Study the drawing (mm; zero at the part's minimum x, y, z) and answer. A direction names the side the tool comes from. Round coordinates to 2 decimals unless told otherwise and drop trailing zeros. Order: outer loops, then holes, each group sorted by start corner. A loop starts at its lowest first (then second) coordinate and runs counter-clockwise, first axis right, second up. Notation, with made-up numbers: (-29.5, 51.5) - (11.5, 51.5) arc R17 ccw to (11.5, 55.5) - close; hole circle Ø9 at (50.5, 43). An arc over 180 degrees is marked (long way). Put each result on its own line as item: value. Start each with the question number.
Q1. Section C-C on x = 3.5 is taken. Give the vertices of the cut face in (y, z) (3 decimals).
Q2. Section B-B on y = 17 is taken. Give the vertices of the cut face in (x, z), then the cut area to 3 significant figures.
Q3. Each of these flat-tipped pins is pushed along its axis until it touches: pin 1 Ø8 at (x, z) = (7, 14) entering from +Y; pin 2 Ø8.5 at (y, z) = (15, 15) entering from +X; pin 3 Ø6 at (y, z) = (15, 15) entering from -X; pin 4 Ø5 at (x, z) = (11.5, 19) entering from +Y. Where does it stop, or does it pass through?
Q4. Find the intervals of material crossed by line 1 along Z through (x, y) = (8.75, 15) (3 decimals); line 2 along Z through (x, y) = (19, 19.25); line 3 along Y through (x, z) = (5.25, 14), in increasing order. Write a range as from..to.
Q5. Section D-D on z = 7 is taken. Give the vertices of the cut face in (x, y).
Q6. For a pull along Y with two mould halves and no side action, classify the marked faces 1, 2 and 3 as pulls with the +Y half, pulls with the -Y half, needs draft (parallel to the pull), parting line crosses it, or undercut.
Q7. Which of the six approach directions +Z, -Z, +X, -X, +Y, -Y give full straight-line access (tool end or side, diameter ignored) to the marked faces 4 and 5?
Q8. Section A-A on z = 15 is taken. Give the vertices of the cut face in (x, y) (3 decimals), then the cut area to 3 significant figures.
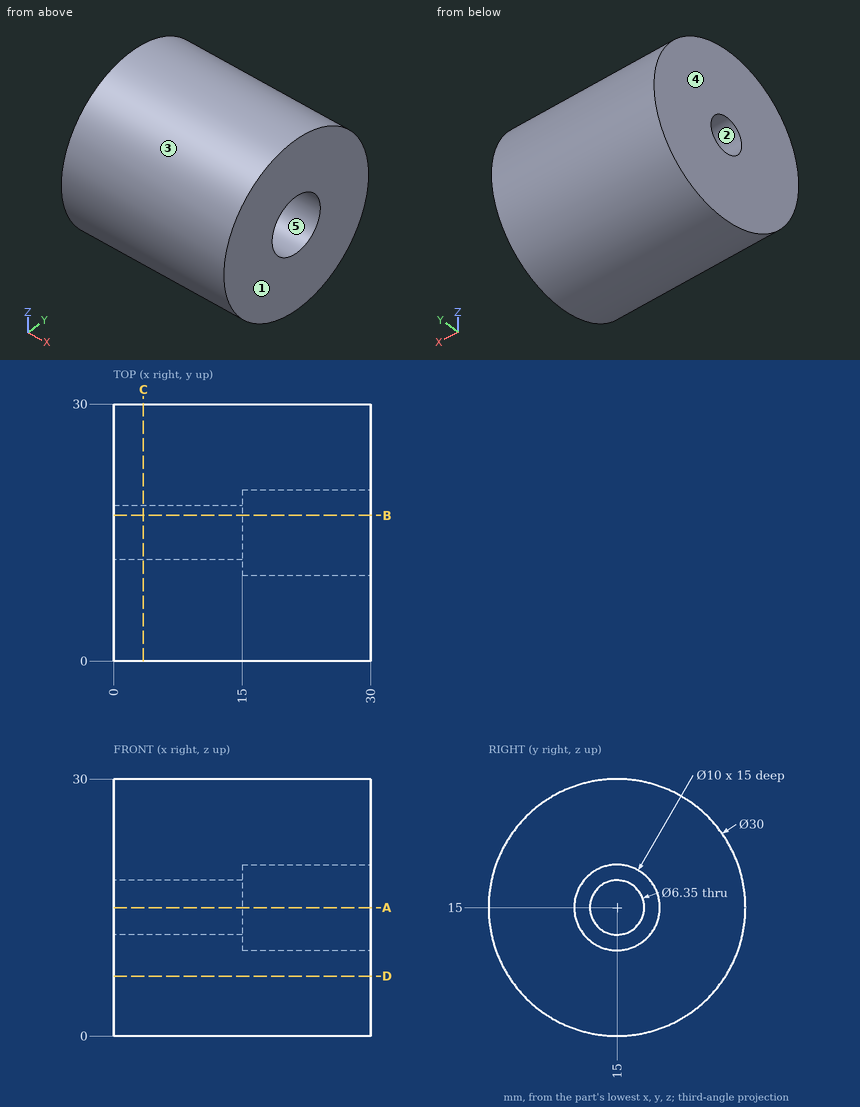
Findings:
1. outline: circle Ø30 at (15, 15); hole circle Ø6.35 at (15, 15)
2. outline: (0, 0.13) - (30, 0.13) - (30, 10.42) - (15, 10.42) - (15, 12.53) - (0, 12.53) - close; (0, 17.47) - (15, 17.47) - (15, 19.58) - (30, 19.58) - (30, 29.87) - (0, 29.87) - close
2. area: 681 mm2
3. pin 1: y = 30
3. pin 2: x = 15
3. pin 3: through
3. pin 4: y = 29.92
4. line 1: 0..11.825, 18.175..30
4. line 2: 0.61..12.37, 17.63..29.39
4. line 3: 0.03..11.99, 18.01..29.97
5. outline: (0, 2.31) - (30, 2.31) - (30, 27.69) - (0, 27.69) - close
6. face 1: needs draft
6. face 2: undercut
6. face 3: parting line crosses it
7. face 4: +Z, -Z, -X, +Y, -Y
7. face 5: +X
8. outline: (0, 0) - (30, 0) - (30, 10) - (15, 10) - (15, 11.825) - (0, 11.825) - close; (0, 18.175) - (15, 18.175) - (15, 20) - (30, 20) - (30, 30) - (0, 30) - close
8. area: 655 mm2
